Geometry check sheet. Reference: the model listing, model coordinates, mm. A direction names the side the tool comes from. Coordinates: 2 decimals unless noted, no trailing zeros. Loops run counter-clockwise (first coordinate to the right, second up) from the corner with the lowest first, then second, coordinate; pieces in that order, holes last. Notation, with made-up numbers: (75.25, 42) -> (84.25, 42) arc R7 cw to (84.25, 50) -> close; hole circle Ø10 at (57.5, 87). An arc over 180 degrees is marked (long way). Answer as a JSON object with one key per item and string values.
from build123d import *

# Parameters (mm, degrees)
SKETCH_1_R          = 11
SKETCH_1_R_2        = 1.75
EXTRUDE_1_DEPTH     = 3
SKETCH_2_R          = 7.5
EXTRUDE_2_DEPTH     = 16
SKETCH_10_W         = 2.3
SKETCH_10_H         = 5.3
CUT_EXTRUDE_4_DEPTH = 16
CUT_EXTRUDE_START   = -16
CUT_EXTRUDE_5_DEPTH = 16
SKETCH_13_R         = 2.7
CUT_EXTRUDE_6_DEPTH = 8
FILLET_1_R          = 1
SKETCH_15_R         = 1.75
CUT_EXTRUDE_7_DEPTH = 10


with BuildPart() as part:
    # 草图1 → 凸台-拉伸1 (new body)
    with BuildSketch(Plane.XY):
        Circle(SKETCH_1_R)
        with Locations((0, 7)):
            Circle(SKETCH_1_R_2, mode=Mode.SUBTRACT)
        with Locations((7, 0)):
            Circle(SKETCH_1_R_2, mode=Mode.SUBTRACT)
        with Locations((0, -7)):
            Circle(SKETCH_1_R_2, mode=Mode.SUBTRACT)
        with Locations((-7, 0)):
            Circle(SKETCH_1_R_2, mode=Mode.SUBTRACT)
    extrude(amount=EXTRUDE_1_DEPTH)

    # 草图2 → 凸台-拉伸2 (add)
    with BuildSketch(Plane.XY.offset(3)):
        with Locations(Location((0, 0, 0), (0, 0, 166.708822757))):
            Circle(SKETCH_2_R)
        with BuildLine():
            Line((-2, 1.738533865), (-2, -1.738533865))
            ThreePointArc((-2, -1.738533865), (-1.295035867, -2.31200824), (-0.437775279, -2.613590022))
            ThreePointArc((-0.437775279, -2.613590022), (2.018459157, -1.717068034), (2.50959842, 0.851126176))
            ThreePointArc((2.50959842, 0.851126176), (0.511659788, 2.600135431), (-2, 1.738533865))
        make_face(mode=Mode.SUBTRACT)
    extrude(amount=EXTRUDE_2_DEPTH)

    # 草图10 → 切除-拉伸4 (cut)
    with BuildSketch(Plane.XY.offset(19)):
        with Locations((-4.65, 0)):
            Rectangle(SKETCH_10_W, SKETCH_10_H)
    extrude(amount=-CUT_EXTRUDE_4_DEPTH, mode=Mode.SUBTRACT)

    # 草图12 → 切除-拉伸5 (cut)
    with BuildSketch(Plane.XY.offset(19).offset(CUT_EXTRUDE_START)):
        with BuildLine():
            Line((-5.452293096, 5.15), (4, 5.15))
            Line((4, 5.15), (4, -5.15))
            Line((4, -5.15), (-5.452293096, -5.15))
            ThreePointArc((-5.452293096, -5.15), (7.5, 0), (-5.452293096, 5.15))
        make_face()
    extrude(amount=CUT_EXTRUDE_5_DEPTH, mode=Mode.SUBTRACT)

    # 草图13 → 切除-拉伸6 (cut)
    with BuildSketch(Plane.XY.offset(3)):
        with Locations((0, 7)):
            Circle(SKETCH_13_R)
        with Locations((7, 0)):
            Circle(SKETCH_13_R)
        with Locations((0, -7)):
            Circle(SKETCH_13_R)
        with Locations((-7, 0)):
            Circle(SKETCH_13_R)
    extrude(amount=CUT_EXTRUDE_6_DEPTH, mode=Mode.SUBTRACT)

    # 圆角1
    # the kernel refuses this fillet: 1 mm, written as the material it adds along each edge
    with BuildSketch(Plane(origin=(0, 0, 3), x_dir=(-0.46227667345108353, 0.8867357425879484, 0), z_dir=(0.8867357425879484, 0.46227667345108353, 0))) as fillet_1_piece_1_section:
        with BuildLine():
            CenterArc((7.5 + FILLET_1_R, FILLET_1_R), FILLET_1_R, 180, 90)
            Line((7.5, FILLET_1_R), (7.5, 0))
            Line((7.5, 0), (7.5 + FILLET_1_R, 0))
        make_face()
    fillet_1_piece_1 = revolve(axis=Axis((0, 0, 3), (0, 0, 1)), revolution_arc=60.46476408, mode=Mode.PRIVATE)
    fillet_1_piece_1 = fillet_1_piece_1 - Plane(origin=(-7, 0, 3.226381538), x_dir=(1, 0, 0), z_dir=(0, 0, -1)) * Cylinder(2.7, 34, mode=Mode.PRIVATE)
    fillet_1_piece_1 = split(fillet_1_piece_1, bisect_by=Plane(origin=(-6.580020659, 5.15, 3.226381538), z_dir=(0, -1, 0)), keep=Keep.TOP, mode=Mode.PRIVATE)
    add(fillet_1_piece_1)
    with BuildSketch(Plane(origin=(0.533403956, -5.15, 3), x_dir=(0, -1, 0), z_dir=(-1, 0, 0))) as fillet_1_piece_2_section:
        with BuildLine():
            CenterArc((FILLET_1_R, FILLET_1_R), FILLET_1_R, 180, 90)
            Line((0, FILLET_1_R), (0, 0))
            Line((0, 0), (FILLET_1_R, 0))
        make_face()
    fillet_1_piece_2 = extrude(amount=8.485697052, mode=Mode.PRIVATE)
    fillet_1_piece_2 = fillet_1_piece_2 - Plane(origin=(0, -7, 3.242251881), x_dir=(1, 0, 0), z_dir=(0, 0, -1)) * Cylinder(2.7, 21, mode=Mode.PRIVATE)
    fillet_1_piece_2 = fillet_1_piece_2 & Plane(origin=(0, 0, 3.242251881), x_dir=(-0.9732142857144194, 0.2298998783848582, 0), z_dir=(0, 0, -1)) * Cylinder(7.5, 21, mode=Mode.PRIVATE)
    add(fillet_1_piece_2)
    with BuildSketch(Plane(origin=(-7.952293096, 5.15, 3), x_dir=(0, 1, 0), z_dir=(1, 0, 0))) as fillet_1_piece_3_section:
        with BuildLine():
            CenterArc((FILLET_1_R, FILLET_1_R), FILLET_1_R, 180, 90)
            Line((0, FILLET_1_R), (0, 0))
            Line((0, 0), (FILLET_1_R, 0))
        make_face()
    fillet_1_piece_3 = extrude(amount=8.485697052, mode=Mode.PRIVATE)
    fillet_1_piece_3 = fillet_1_piece_3 - Plane(origin=(0, 7, 3.242252003), x_dir=(1, 0, 0), z_dir=(0, 0, -1)) * Cylinder(2.7, 21, mode=Mode.PRIVATE)
    fillet_1_piece_3 = fillet_1_piece_3 & Plane(origin=(0, 0, 3.242252003), x_dir=(-0.9732142857144194, 0.2298998783848582, 0), z_dir=(0, 0, -1)) * Cylinder(7.5, 21, mode=Mode.PRIVATE)
    add(fillet_1_piece_3)
    with BuildSketch(Plane(origin=(0, 0, 3), x_dir=(-0.9993901440206632, -0.034919049734468105, 0), z_dir=(-0.034919049734468105, 0.9993901440206632, 0))) as fillet_1_piece_4_section:
        with BuildLine():
            CenterArc((7.5 + FILLET_1_R, FILLET_1_R), FILLET_1_R, 180, 90)
            Line((7.5, FILLET_1_R), (7.5, 0))
            Line((7.5, 0), (7.5 + FILLET_1_R, 0))
        make_face()
    fillet_1_piece_4 = revolve(axis=Axis((0, 0, 3), (0, 0, 1)), revolution_arc=60.46476408, mode=Mode.PRIVATE)
    fillet_1_piece_4 = fillet_1_piece_4 - Plane(origin=(-7, 0, 3.226381502), x_dir=(1, 0, 0), z_dir=(0, 0, -1)) * Cylinder(2.7, 35, mode=Mode.PRIVATE)
    fillet_1_piece_4 = split(fillet_1_piece_4, bisect_by=Plane(origin=(-6.580021181, -5.15, 3.226381502), z_dir=(0, 1, 0)), keep=Keep.TOP, mode=Mode.PRIVATE)
    add(fillet_1_piece_4)
    with BuildSketch(Plane(origin=(0, 0, 3), x_dir=(-0.46227667345108353, 0.8867357425879484, 0), z_dir=(0.8867357425879484, 0.46227667345108353, 0))) as fillet_1_piece_5a_section:
        with BuildLine():
            CenterArc((7.5 + FILLET_1_R, FILLET_1_R), FILLET_1_R, 180, 90)
            Line((7.5, FILLET_1_R), (7.5, 0))
            Line((7.5, 0), (7.5 + FILLET_1_R, 0))
        make_face()
    fillet_1_piece_5a = revolve(axis=Axis((0, 0, 3), (0, 0, 1)), revolution_arc=60.46476408, mode=Mode.PRIVATE)
    fillet_1_piece_5a = split(fillet_1_piece_5a, bisect_by=Plane(origin=(-4.735225186, 5.15, 3.214069689), z_dir=(0, 1, 0)), keep=Keep.TOP, mode=Mode.PRIVATE)
    with BuildSketch(Plane(origin=(-7.952293096, 5.15, 3), x_dir=(0, 1, 0), z_dir=(1, 0, 0))) as fillet_1_piece_5b_section:
        with BuildLine():
            CenterArc((FILLET_1_R, FILLET_1_R), FILLET_1_R, 180, 90)
            Line((0, FILLET_1_R), (0, 0))
            Line((0, 0), (FILLET_1_R, 0))
        make_face()
    fillet_1_piece_5b = extrude(amount=8.485697052, mode=Mode.PRIVATE)
    fillet_1_piece_5b = fillet_1_piece_5b - Plane(origin=(0, 0, 3.215737548), x_dir=(-0.9732142857144194, 0.2298998783848582, 0), z_dir=(0, 0, -1)) * Cylinder(7.5, 21, mode=Mode.PRIVATE)
    fillet_1_piece_5 = fillet_1_piece_5a & fillet_1_piece_5b
    add(fillet_1_piece_5)
    with BuildSketch(Plane(origin=(0.533403956, -5.15, 3), x_dir=(0, -1, 0), z_dir=(-1, 0, 0))) as fillet_1_piece_6a_section:
        with BuildLine():
            CenterArc((FILLET_1_R, FILLET_1_R), FILLET_1_R, 180, 90)
            Line((0, FILLET_1_R), (0, 0))
            Line((0, 0), (FILLET_1_R, 0))
        make_face()
    fillet_1_piece_6a = extrude(amount=8.485697052, mode=Mode.PRIVATE)
    fillet_1_piece_6a = fillet_1_piece_6a - Plane(origin=(0, 0, 3.215737542), x_dir=(-0.9732142857144194, 0.2298998783848582, 0), z_dir=(0, 0, -1)) * Cylinder(7.5, 21, mode=Mode.PRIVATE)
    with BuildSketch(Plane(origin=(0, 0, 3), x_dir=(-0.9993901440206632, -0.034919049734468105, 0), z_dir=(-0.034919049734468105, 0.9993901440206632, 0))) as fillet_1_piece_6b_section:
        with BuildLine():
            CenterArc((7.5 + FILLET_1_R, FILLET_1_R), FILLET_1_R, 180, 90)
            Line((7.5, FILLET_1_R), (7.5, 0))
            Line((7.5, 0), (7.5 + FILLET_1_R, 0))
        make_face()
    fillet_1_piece_6b = revolve(axis=Axis((0, 0, 3), (0, 0, 1)), revolution_arc=60.46476408, mode=Mode.PRIVATE)
    fillet_1_piece_6b = split(fillet_1_piece_6b, bisect_by=Plane(origin=(-4.735225263, -5.15, 3.214069799), z_dir=(0, -1, 0)), keep=Keep.TOP, mode=Mode.PRIVATE)
    fillet_1_piece_6 = fillet_1_piece_6a & fillet_1_piece_6b
    add(fillet_1_piece_6)
    # the kernel refuses this fillet: 1 mm, written as the material it takes off along each edge
    with BuildSketch(Plane(origin=(4, -5.15, 3), x_dir=(-1, 0, 0), z_dir=(0, 0, 1)), Plane(origin=(4, 5.15, 3), x_dir=(0, -1, 0), z_dir=(0, 0, 1))) as fillet_1_2_piece_1:
        with BuildLine():
            CenterArc((FILLET_1_R, -FILLET_1_R), FILLET_1_R, 90, 90)
            Line((0, -FILLET_1_R), (0, 0))
            Line((0, 0), (FILLET_1_R, 0))
        make_face()
    extrude(amount=18.5, mode=Mode.SUBTRACT)
    # the kernel refuses this fillet: 1 mm, written as the material it adds along each edge
    with BuildSketch(Plane(origin=(4, 4.15, 3), x_dir=(1, 0, 0), z_dir=(0, -1, 0))) as fillet_1_3_piece_1:
        with BuildLine():
            CenterArc((FILLET_1_R, FILLET_1_R), FILLET_1_R, 180, 90)
            Line((0, FILLET_1_R), (0, 0))
            Line((0, 0), (FILLET_1_R, 0))
        make_face()
    extrude(amount=8.3)
    with BuildSketch(Plane(origin=(-0.533403956, 5.15, 3), x_dir=(0, 1, 0), z_dir=(1, 0, 0))) as fillet_1_3_piece_2_section:
        with BuildLine():
            CenterArc((FILLET_1_R, FILLET_1_R), FILLET_1_R, 180, 90)
            Line((0, FILLET_1_R), (0, 0))
            Line((0, 0), (FILLET_1_R, 0))
        make_face()
    fillet_1_3_piece_2 = extrude(amount=3.533403956, mode=Mode.PRIVATE)
    fillet_1_3_piece_2 = fillet_1_3_piece_2 - Plane(origin=(0, 7, 3.249320301), x_dir=(1, 0, 0), z_dir=(0, 0, -1)) * Cylinder(2.7, 12, mode=Mode.PRIVATE)
    add(fillet_1_3_piece_2)
    with BuildSketch(Plane(origin=(3, -5.15, 3), x_dir=(0, -1, 0), z_dir=(-1, 0, 0))) as fillet_1_3_piece_3_section:
        with BuildLine():
            CenterArc((FILLET_1_R, FILLET_1_R), FILLET_1_R, 180, 90)
            Line((0, FILLET_1_R), (0, 0))
            Line((0, 0), (FILLET_1_R, 0))
        make_face()
    fillet_1_3_piece_3 = extrude(amount=3.533403956, mode=Mode.PRIVATE)
    fillet_1_3_piece_3 = fillet_1_3_piece_3 - Plane(origin=(0, -7, 3.249320301), x_dir=(1, 0, 0), z_dir=(0, 0, -1)) * Cylinder(2.7, 12, mode=Mode.PRIVATE)
    add(fillet_1_3_piece_3)
    with BuildSketch(Plane(origin=(3, -4.15, 3), x_dir=(0, -1, 0), z_dir=(-1, 0, 0))) as fillet_1_3_piece_4:
        with BuildLine():
            CenterArc((1 + FILLET_1_R, FILLET_1_R), FILLET_1_R, 180, 90)
            Line((1, FILLET_1_R), (1, 0))
            Line((1, 0), (1 + FILLET_1_R, 0))
        make_face()
    revolve(axis=Axis((3, -4.15, 3), (0, 0, 1)), revolution_arc=90)
    with BuildSketch(Plane(origin=(3, 4.15, 3), x_dir=(1, 0, 0), z_dir=(0, -1, 0))) as fillet_1_3_piece_5:
        with BuildLine():
            CenterArc((1 + FILLET_1_R, FILLET_1_R), FILLET_1_R, 180, 90)
            Line((1, FILLET_1_R), (1, 0))
            Line((1, 0), (1 + FILLET_1_R, 0))
        make_face()
    revolve(axis=Axis((3, 4.15, 3), (0, 0, 1)), revolution_arc=90)

    # 草图15 → 切除-拉伸7 (cut)
    with BuildSketch(Plane(origin=(-10.8, 0, 0), x_dir=(0, 0, -1), z_dir=(1, 0, 0))):
        with Locations(Location((-14.5, 0, 0), (0, 0, 263.437572131))):
            Circle(SKETCH_15_R)
    extrude(amount=CUT_EXTRUDE_7_DEPTH, mode=Mode.SUBTRACT)


solid = part.part
1. Section check C-C, the plane z = 2.25. Record the boundary of the cut face in (x, y).
Evaluation:
{"outline": "circle Ø22 at (0, 0); hole circle Ø3.5 at (-7, 0); hole circle Ø3.5 at (0, -7); hole circle Ø3.5 at (0, 7); hole circle Ø3.5 at (7, 0)"}
2. Tool access check on faces 1 (the face through (4, 0, 11)), 2 (the face through (3.699, -4.865, 11.395)), 3 (the face through (0, 5, 11)). Record the directions out of +Z, -Z, +X, -X, +Y, -Y that give a thin tool (end or side, any length) a straight path to the whole face; none if there is none.
Evaluation:
{"face 1": "+Z, +X, +Y, -Y", "face 2": "+Z, +X, -Y", "face 3": "+Y"}
3. Thickness scan on probe 1 along Y at (x, z) = (-2.75, 14.5); probe 2 along Z at (x, y) = (-2.55, 0); probe 3 along Z at (x, y) = (-4, 0). Record the ranges inside material, lowest first. Write a range as from..to.
Evaluation:
{"probe 1": "y = -5.15..-1.75, 1.75..5.15", "probe 2": "z = 0..12.75, 16.25..19", "probe 3": "z = 0..3"}
4. Section check A-A, the plane y = 0. State how many separate pieces and enclosed holes the cut face has, then the cut area to 3 significant figures.
Evaluation:
{"separate pieces": "6", "enclosed holes": "0", "area": "93.2 mm^2"}
5. Depth check by flat-ended pin: P1, Ø4, axis at x = -5.5, z = 14.5, coming from the +Y side; P2, Ø1.8, axis at x = -4.5, z = 9.5, coming from the -Y side; P3, Ø1.4, axis at x = 1, y = 1, coming from the +Z side; P4, Ø3, axis at x = 0, y = 7, coming from the -Z side. Enter the tip coordinate at first touch or a pass-through.
Evaluation:
{"P1": "stops at y = 5.15", "P2": "stops at y = -5.15", "P3": "stops at z = 3", "P4": "passes through"}
6. Mould release check, pull along Y, two halves, no side actions. Record for faces 4 (the face through (0, 0, 0)), 5 (the face through (-6.7, -1.5, 15.4)), 6 (the face through (-2.38, -10.74, 1.48)): released by +Y, released by -Y, zero draft, split by the parting line, or undercut.
Evaluation:
{"face 4": "zero draft", "face 5": "undercut", "face 6": "split by the parting line"}
7. Section check B-B, the plane x = 0. Record the boundary of the cut face in (y, z).
Evaluation:
{"outline": "(-11, 0) -> (-8.75, 0) -> (-8.75, 3) -> (-11, 3) -> close; (-5.25, 0) -> (5.25, 0) -> (5.25, 3) -> (4.3, 3) -> (4.3, 11) -> (5.15, 11) -> (5.15, 19) -> (2.65, 19) -> (2.65, 3) -> (-2.65, 3) -> (-2.65, 19) -> (-5.15, 19) -> (-5.15, 11) -> (-4.3, 11) -> (-4.3, 3) -> (-5.25, 3) -> close; (8.75, 0) -> (11, 0) -> (11, 3) -> (8.75, 3) -> close"}
8. Section check D-D, the plane z = 17. Record the boundary of the cut face in (x, y), then the cut area to 3 significant figures.
Evaluation:
{"outline": "(-5.45, -5.15) -> (3, -5.15) arc R1 ccw to (4, -4.15) -> (4, 4.15) arc R1 ccw to (3, 5.15) -> (-5.45, 5.15) arc R7.5 ccw to start; hole (-5.8, -2.65) -> (-3.5, -2.65) -> (-3.5, 2.65) -> (-5.8, 2.65) -> close; hole (-2, -1.74) arc R2.65 ccw (long way) to (-2, 1.74) -> close", "area": "78.7 mm^2"}
